Geometry: see drawing. Coordinates: mm, zero at the bounding-box minimum. A direction names the side the tool comes from. Give positions to 0.01 mm unless a question says otherwise; leave off trailing zeros. Write each loop counter-clockwise with the first axis right and the second up, starting at its lowest first coordinate (ties: lowest second). Pieces come first, ordered by that corner, then holes. Notation, with made-up numbers: (26.25, -8) - (57.25, -8) arc R12 cw to (57.25, 13) - close; hole circle Ø4 at (-24.75, 6.5). An arc over 180 degrees is marked (long way). Answer as CSV lines item,"result". Start each with the question number.
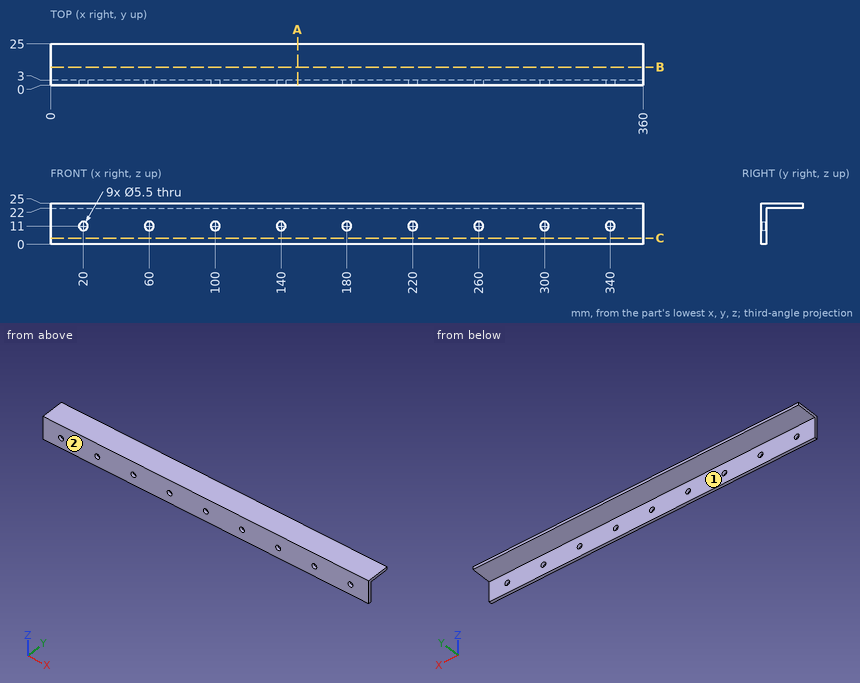
1) Material intervals for line 1 (Z direction, x = 220, y = 2.05); line 2 (Z direction, x = 123.5, y = 7); line 3 (Y direction, x = 201, z = 4.25), sorted ascending. Write a range as from..to.
2) Reachability of the marked faces 1 and 2 from +Z, -Z, +X, -X, +Y, -Y: full face, straight path, thin tool, end or side. Return the list, or none.
3) Cut plane A-A on x = 150. Output: boundary loops of the cut face in (y, z).
4) Cut plane B-B on y = 11. Output: boundary loops of the cut face in (x, z), and give its area (3 significant figures).
5) Cut plane C-C on z = 3.75. Output: boundary loops of the cut face in (x, y), and give its area (3 significant figures).
6) Contact query for flat-ended pins moving along their axis: P1, Ø6.5, axis at x = 210, y = 12, coming from the -Z side; P2, Ø4, axis at x = 285.5, z = 20, coming from the -Y side; P3, Ø7, axis at x = 100, z = 11, coming from the +Y side. Output: stop coordinate, or through.
Numbers:
1,line 1,"z = 0..8.25, 13.75..25"
1,line 2,"z = 22..25"
1,line 3,"y = 0..3"
2,face 1,"-Z, +X, -X, +Y"
2,face 2,"+Z, -Z, +X, -X, -Y"
3,outline,"(0, 0) - (3, 0) - (3, 22) - (25, 22) - (25, 25) - (0, 25) - close"
4,outline,"(0, 22) - (360, 22) - (360, 25) - (0, 25) - close"
4,area,"1,080 mm²"
5,outline,"(0, 0) - (360, 0) - (360, 3) - (0, 3) - close"
5,area,"1,080 mm²"
6,P1,"stops at z = 22"
6,P2,"stops at y = 0"
6,P3,"stops at y = 3"
